Check sheet for the modelled part. Datum: model origin and axes. Units: mm. Face numbers are marked on the shaded views. A direction names the side the tool comes from. Round coordinates to 2 decimals unless told otherwise and drop trailing zeros. Loops run counter-clockwise (first coordinate to the right, second up) from the corner with the lowest first, then second, coordinate; pieces in that order, holes last. Notation, with made-up numbers: (-32.75, -0.5) -> (-20.75, -0.5) arc R23 ccw to (-20.75, 22.5) -> close; hole circle Ø3 at (35, -32). An arc over 180 degrees is marked (long way). One line per item, written item: value. Start each with the question number.
1. Cross-section at A-A on z = 0. Record the cut outline in (x, y) (3 decimals).
2. Go/stop test with flat-tipped pins: pin 1 (5 mm diameter, centred on x = 4.5, y = 15, fed in from +Z); pin 2 (1.5 mm diameter, centred on x = 0, y = 104.53, fed in from +Z); pin 3 (3 mm diameter, centred on x = -11.5, y = 32.5, fed in from +Z). Record where each tip stops, or that it passes through.
3. Set-up check for the marked faces 1, 2 and 3: record each of +Z, -Z, +X, -X, +Y, -Y from which the full face is reachable in a straight line by a thin tool's end or side.
4. Cross-section at C-C on y = 11. Record the cut outline in (x, z), then the cut area to 3 significant figures.
5. Material ranges on L1, parallel to Y at x = -0.5, z = -19; L2, parallel to X at y = 38, z = 12.5; L3, parallel to X at y = 45, z = -19.5, recorded low to high.
6. Cross-section at B-B on y = 75. Record the cut outline in (x, z) (3 decimals).
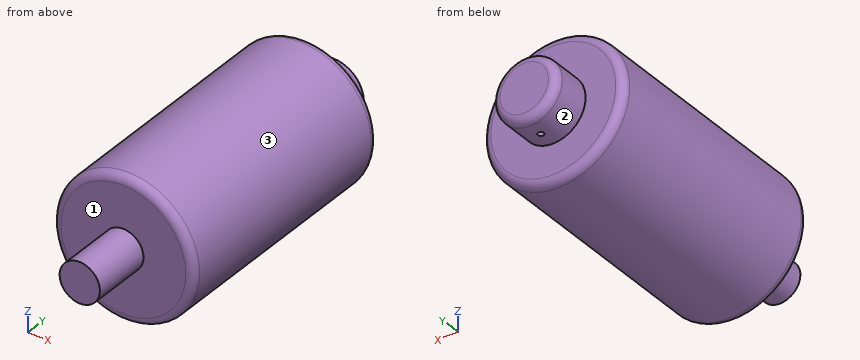
from build123d import *

# Parameters (mm, degrees)
SKETCH1_R           = 6.35
BOSS_EXTRUDE1_DEPTH = 19.05
SKETCH3_R           = 22.225
BOSS_EXTRUDE2_DEPTH = 80.01
SKETCH4_R           = 10.16
BOSS_EXTRUDE3_DEPTH = 12.7
FILLET2_R           = 2.54
FILLET3_R           = 2.54
FILLET4_R           = 2.54
SKETCH5_R           = 0.948603759
CUT_EXTRUDE1_DEPTH  = 2.54


with BuildPart() as part:
    # Sketch1 → Boss-Extrude1 (new body)
    with BuildSketch(Plane(origin=(0, 0, 0), x_dir=(1, 0, 0), z_dir=(0, 1, 0))):
        with Locations(Location((0, 0, 0), (0, 0, 90))):
            Circle(SKETCH1_R)
    extrude(amount=BOSS_EXTRUDE1_DEPTH)

    # Sketch3 → Boss-Extrude2 (add)
    with BuildSketch(Plane(origin=(0, 19.05, 0), x_dir=(1, 0, 0), z_dir=(0, 1, 0))):
        with Locations(Location((0, 0, 0), (0, 0, 270))):
            Circle(SKETCH3_R)
    extrude(amount=BOSS_EXTRUDE2_DEPTH)

    # Sketch4 → Boss-Extrude3 (add)
    with BuildSketch(Plane(origin=(0, 99.06, 0), x_dir=(1, 0, 0), z_dir=(0, 1, 0))):
        with Locations(Location((0, 0, 0), (0, 0, 270))):
            Circle(SKETCH4_R)
    extrude(amount=BOSS_EXTRUDE3_DEPTH)

    # Fillet2
    fillet2_edges = [part.edges().sort_by_distance(p)[0] for p in [
        (0, 111.76, -10.16),
    ]]
    fillet(fillet2_edges, radius=FILLET2_R)

    # Fillet3
    fillet3_edges = [part.edges().sort_by_distance(p)[0] for p in [
        (0, 99.06, -22.225),
    ]]
    fillet(fillet3_edges, radius=FILLET3_R)

    # Fillet4
    fillet4_edges = [part.edges().sort_by_distance(p)[0] for p in [
        (0, 19.05, -22.225),
    ]]
    fillet(fillet4_edges, radius=FILLET4_R)

    # Sketch5 → Cut-Extrude1 (cut)
    with BuildSketch(Plane(origin=(0, 0, -10.16), x_dir=(-1, 0, 0), z_dir=(0, 0, -1))):
        with Locations((0, 104.531305945)):
            Circle(SKETCH5_R)
    extrude(amount=-CUT_EXTRUDE1_DEPTH, mode=Mode.SUBTRACT)


solid = part.part
Taken from the geometry:
1. outline: (-22.225, 21.59) arc R2.54 ccw to (-19.685, 19.05) -> (-6.35, 19.05) -> (-6.35, 0) -> (6.35, 0) -> (6.35, 19.05) -> (19.685, 19.05) arc R2.54 ccw to (22.225, 21.59) -> (22.225, 96.52) arc R2.54 ccw to (19.685, 99.06) -> (10.16, 99.06) -> (10.16, 109.22) arc R2.54 ccw to (7.62, 111.76) -> (-7.62, 111.76) arc R2.54 ccw to (-10.16, 109.22) -> (-10.16, 99.06) -> (-19.685, 99.06) arc R2.54 ccw to (-22.225, 96.52) -> close
2. pin 1: stops at z = 6.03
2. pin 2: stops at z = 10.16
2. pin 3: stops at z = 19.85
3. face 1: -Y
3. face 2: +Y
3. face 3: +Y, -Y
4. outline: circle Ø12.7 at (0, 0)
4. area: 127 mm2
5. L1: y = 19.05 to 99.06
5. L2: x = -18.38 to 18.38
5. L3: x = -10.66 to 10.66
6. outline: circle Ø44.45 at (0, 0)
